Build history of the part. All positions in model axes, mm. A direction names the side the tool comes from. Give positions to 0.01 mm unless a question says otherwise; leave off trailing zeros. Order: outer loops, then holes, each group sorted by start corner. A loop starts at its lowest first (then second) coordinate and runs counter-clockwise, first axis right, second up. Notation, with made-up numbers: M 67,29.25 L 90,29.25 A24 ccw 90,55.25 Z; hole C 66.5,-29 d5. An arc over 180 degrees is marked long. One line per item, written item: value.
from build123d import *

# Parameters (mm, degrees)
ESQUISSE1_R             = 13
ESQUISSE1_R_2           = 5.5
BOSS_EXTRU_1_DEPTH      = 8
ESQUISSE2_W             = 32.31004566
ESQUISSE2_H             = 49.818141682
ENL_V_MAT_EXTRU_1_DEPTH = 8
ESQUISSE3_R             = 1.5
ENL_V_MAT_EXTRU_2_DEPTH = 8
ESQUISSE4_W             = 24.87123002
ESQUISSE4_H             = 13.833010023
ESQUISSE4_W_2           = 23.432073676
ESQUISSE4_H_2           = 10.309386407
ENL_V_MAT_EXTRU_3_DEPTH = 8
ENL_V_MAT_EXTRU_4_DEPTH = 8
ESQUISSE7_W             = 3
ESQUISSE7_H             = 5.75
BOSS_EXTRU_3_DEPTH      = 8
ESQUISSE11_R            = 1.5
ENL_V_MAT_EXTRU_5_DEPTH = 8
CONG_5_R                = 0.5
CONG_6_R                = 0.5
CONG_7_R                = 0.5
CONG_8_R                = 0.5


with BuildPart() as part:
    # Esquisse1 → Boss.-Extru.1 (new body)
    with BuildSketch(Plane.XY):
        Circle(ESQUISSE1_R)
        Circle(ESQUISSE1_R_2, mode=Mode.SUBTRACT)
    extrude(amount=BOSS_EXTRU_1_DEPTH)

    # Esquisse2 → Enlèv. mat.-Extru.1 (cut)
    with BuildSketch(Plane.XY.offset(8)):
        with Locations((15.15502283, -0.665904075)):
            Rectangle(ESQUISSE2_W, ESQUISSE2_H)
    extrude(amount=-ENL_V_MAT_EXTRU_1_DEPTH, mode=Mode.SUBTRACT)

    # Esquisse3 → Enlèv. mat.-Extru.2 (cut)
    with BuildSketch(Plane(origin=(-1, 0, 0), x_dir=(0, 0, -1), z_dir=(1, 0, 0))):
        with Locations((-4, 10.461481397)):
            Circle(ESQUISSE3_R)
        with Locations((-4, -10.461481397)):
            Circle(ESQUISSE3_R)
    extrude(amount=-ENL_V_MAT_EXTRU_2_DEPTH, mode=Mode.SUBTRACT)

    # Esquisse4 → Enlèv. mat.-Extru.3 (cut)
    with BuildSketch(Plane.XY.offset(8)):
        with Locations((-16.43561501, 14.127986408)):
            Rectangle(ESQUISSE4_W, ESQUISSE4_H)
        with Locations((-15.716036838, -12.366174601)):
            Rectangle(ESQUISSE4_W_2, ESQUISSE4_H_2)
    extrude(amount=-ENL_V_MAT_EXTRU_3_DEPTH, mode=Mode.SUBTRACT)

    # Esquisse6 → Enlèv. mat.-Extru.4 (cut)
    with BuildSketch(Plane.XY.offset(8)):
        with BuildLine():
            Line((-14.689217928, -10.049334481), (-4.81866764, -7.601344761))
            ThreePointArc((-4.81866764, -7.601344761), (-8.998001154, 0.189671363), (-4.494067947, 7.797650498))
            Line((-4.494067947, 7.797650498), (-11.133481596, 10.892455097))
            ThreePointArc((-11.133481596, 10.892455097), (-17.721132871, 1.238220245), (-14.689217928, -10.049334481))
        make_face()
    extrude(amount=-ENL_V_MAT_EXTRU_4_DEPTH, mode=Mode.SUBTRACT)

    # Esquisse7 → Boss.-Extru.3 (add)
    with BuildSketch(Plane(origin=(0, 0, 0), x_dir=(-1, 0, 0), z_dir=(0, 0, -1))):
        with Locations((2.5, 10.086481397)):
            Rectangle(ESQUISSE7_W, ESQUISSE7_H)
        with Locations((2.5, -10.086481397)):
            Rectangle(ESQUISSE7_W, ESQUISSE7_H)
    extrude(amount=-BOSS_EXTRU_3_DEPTH)

    # Esquisse11 → Enlèv. mat.-Extru.5 (cut)
    with BuildSketch(Plane(origin=(-1, 0, 0), x_dir=(0, 0, -1), z_dir=(1, 0, 0))):
        with Locations((-4, 10.461481397)):
            Circle(ESQUISSE11_R)
        with Locations((-4, -10.461481397)):
            Circle(ESQUISSE11_R)
    extrude(amount=-ENL_V_MAT_EXTRU_5_DEPTH, mode=Mode.SUBTRACT)

    # Congé5
    cong_5_edges = [part.edges().sort_by_distance(p)[0] for p in [
        (-4, 12.961481397, 4),
        (-4, -12.961481397, 4),
    ]]
    fillet(cong_5_edges, radius=CONG_5_R)

    # Congé6
    cong_6_edges = [part.edges().sort_by_distance(p)[0] for p in [
        (-4, 7.211481397, 4),
        (-4, -7.211481397, 4),
    ]]
    fillet(cong_6_edges, radius=CONG_6_R)

    # Congé7
    cong_7_edges = [part.edges().sort_by_distance(p)[0] for p in [
        (-1, 12.961481397, 4),
        (-1, -12.961481397, 4),
    ]]
    fillet(cong_7_edges, radius=CONG_7_R)

    # Congé8
    cong_8_edges = [part.edges().sort_by_distance(p)[0] for p in [
        (-5.384657469, 7.211481397, 4),
        (-5.384657469, -7.211481397, 4),
    ]]
    fillet(cong_8_edges, radius=CONG_8_R)


solid = part.part
1) Saw through at C-C, the plane y = 9.75. Write the cut outline in (x, z), then the cut area to 3 significant figures.
Check values:
outline: M -4,0 L -1,0 L -1,2.68 L -4,2.68 Z; M -4,5.32 L -1,5.32 L -1,8 L -4,8 Z
area: 16.1 mm^2
2) Pin check, flat tips, straight feed: pin 1 (2.5 mm diameter, centred on y = 9.5, z = 4.5, fed in from -X); pin 2 (3 mm diameter, centred on x = -7, y = -8, fed in from +Z). Stop position of each tip, or through.
Check values:
pin 1: x = -4
pin 2: through
3) Tool access for faces 1 (the face through (-4, 9, 5)), 2 (the face through (-6, 0, 8)): list every direction of +Z, -Z, +X, -X, +Y, -Y with a clear straight run to the whole face (end or side of a thin tool).
Check values:
face 1: +Z, -Z, -X, +Y
face 2: +Z, +X, -X, +Y, -Y
4) Mould opens along Y. For faces 3 (the face through (-2, 12.961, 4)), 4 (the face through (-2.5, -11, 2.6)), 5 (the face through (-4, -9, 5)), 6 (the face through (-2.479, 9.887, 2.614)) say: released by +Y, released by -Y, zero draft, split by the parting line, or undercut.
Check values:
face 3: released by +Y
face 4: undercut
face 5: zero draft
face 6: undercut
5) Saw through at B-B, the plane x = -2.25. Write the cut outline in (y, z), then the cut area to 3 significant figures.
Check values:
outline: M -12.96,0 L -5.02,0 L -5.02,8 L -12.96,8 Z; M 5.02,0 L 12.96,0 L 12.96,8 L 5.02,8 Z; hole C -10.46,4 d3; hole C 10.46,4 d3
area: 113 mm^2
6) Drill centre lines: probe 1 along Y at (x, z) = (-1.5, 4); probe 2 along Y at (x, z) = (-1.75, 3); probe 3 along Y at (x, z) = (-1.25, 2). Where is each one in solid material? Low to high. Write a range as from..to.
Check values:
probe 1: -12.96..-11.96, -8.96..-5.29, 5.29..8.96, 11.96..12.96
probe 2: -12.96..-11.58, -9.34..-5.21, 5.21..9.34, 11.58..12.96
probe 3: -12.89..-5.36, 5.36..12.89
7) Saw through at A-A, the plane z = 4. Write the cut outline in (x, y).
Check values:
outline: M -5.52,-7.11 A0.5 ccw -5.22,-7.21 L -4.5,-7.21 A0.5 cw -4,-7.71 L -4,-8.96 L -1,-8.96 L -1,-5.41 A5.5 cw -1,5.41 L -1,8.96 L -4,8.96 L -4,7.71 A0.5 cw -4.5,7.21 L -5.22,7.21 A0.5 ccw -5.52,7.11 A9 ccw Z; M -4,-12.46 A0.5 ccw -3.5,-12.96 L -1.5,-12.96 A0.5 ccw -1,-12.46 L -1,-11.96 L -4,-11.96 Z; M -4,11.96 L -1,11.96 L -1,12.46 A0.5 ccw -1.5,12.96 L -3.5,12.96 A0.5 ccw -4,12.46 Z
8) Saw through at D-D, the plane x = -1.25. Write the cut outline in (y, z).
Check values:
outline: M -12.89,0 L -5.36,0 L -5.36,8 L -12.89,8 Z; M 5.36,0 L 12.89,0 L 12.89,8 L 5.36,8 Z; hole C -10.46,4 d3; hole C 10.46,4 d3
